```python
from build123d import *

# Parameters (mm, degrees)
SKETCH1_R           = 1.5
BOSS_EXTRUDE1_DEPTH = 222.5


with BuildPart() as part:
    # Sketch1 → Boss-Extrude1 (new body)
    with BuildSketch(Plane.XY):
        with BuildLine():
            Line((0.997149379, -0.010991612), (4.197149379, -0.010991612))
            ThreePointArc((4.197149379, -0.010991612), (4.409281413, 0.076876353), (4.497149379, 0.289008388))
            Line((4.497149379, 0.289008388), (4.497149379, 0.689008388))
            ThreePointArc((4.497149379, 0.689008388), (4.409281413, 0.901140422), (4.197149379, 0.989008388))
            Line((4.197149379, 0.989008388), (3.197149379, 0.989008388))
            ThreePointArc((3.197149379, 0.989008388), (2.985017344, 1.076876353), (2.897149379, 1.289008388))
            Line((2.897149379, 1.289008388), (2.897149379, 2.057637538))
            ThreePointArc((2.897149379, 2.057637538), (2.920422177, 2.174637797), (2.9866975, 2.273825827))
            Line((2.9866975, 2.273825827), (4.61806835, 3.905196677))
            ThreePointArc((4.61806835, 3.905196677), (4.71725638, 3.971472), (4.834256639, 3.994744798))
            Line((4.834256639, 3.994744798), (10.171514939, 3.994744798))
            ThreePointArc((10.171514939, 3.994744798), (10.288515198, 3.971472), (10.387703228, 3.905196677))
            Line((10.387703228, 3.905196677), (12.019074078, 2.273825827))
            ThreePointArc((12.019074078, 2.273825827), (12.085349401, 2.174637797), (12.1086222, 2.057637538))
            Line((12.1086222, 2.057637538), (12.1086222, 1.289008388))
            ThreePointArc((12.1086222, 1.289008388), (12.020754234, 1.076876353), (11.8086222, 0.989008388))
            Line((11.8086222, 0.989008388), (10.797149379, 0.989008388))
            ThreePointArc((10.797149379, 0.989008388), (10.585017344, 0.901140422), (10.497149379, 0.689008388))
            Line((10.497149379, 0.689008388), (10.497149379, 0.289008388))
            ThreePointArc((10.497149379, 0.289008388), (10.585017344, 0.076876353), (10.797149379, -0.010991612))
            Line((10.797149379, -0.010991612), (13.997149379, -0.010991612))
            ThreePointArc((13.997149379, -0.010991612), (14.70425616, 0.281901607), (14.997149379, 0.989008388))
            Line((14.997149379, 0.989008388), (14.997149379, 4.189008388))
            ThreePointArc((14.997149379, 4.189008388), (14.909281413, 4.401140422), (14.697149379, 4.489008388))
            Line((14.697149379, 4.489008388), (14.305261888, 4.489008388))
            ThreePointArc((14.305261888, 4.489008388), (14.093129854, 4.401140422), (14.005261888, 4.189008388))
            Line((14.005261888, 4.189008388), (14.005261888, 3.189008388))
            ThreePointArc((14.005261888, 3.189008388), (13.917393922, 2.976876353), (13.705261888, 2.889008388))
            Line((13.705261888, 2.889008388), (12.936632738, 2.889008388))
            ThreePointArc((12.936632738, 2.889008388), (12.819632479, 2.912281186), (12.720444449, 2.978556509))
            Line((12.720444449, 2.978556509), (11.089073599, 4.609927359))
            ThreePointArc((11.089073599, 4.609927359), (11.006246661, 4.70520219), (10.969948855, 4.826115648))
            Line((10.969948855, 4.826115648), (10.969948855, 10.163373948))
            ThreePointArc((10.969948855, 10.163373948), (11.00546556, 10.284783861), (11.087867966, 10.380761184))
            Line((11.087867966, 10.380761184), (12.719238816, 12.012132034))
            ThreePointArc((12.719238816, 12.012132034), (12.81656582, 12.07716386), (12.93137085, 12.1))
            Line((12.93137085, 12.1), (13.7, 12.1))
            ThreePointArc((13.7, 12.1), (13.912132034, 12.012132034), (14, 11.8))
            Line((14, 11.8), (14, 10.8))
            ThreePointArc((14, 10.8), (14.087867966, 10.587867966), (14.3, 10.5))
            Line((14.3, 10.5), (14.697149379, 10.5))
            ThreePointArc((14.697149379, 10.5), (14.909281413, 10.587867966), (14.997149379, 10.8))
            Line((14.997149379, 10.8), (14.997149379, 13.989008388))
            ThreePointArc((14.997149379, 13.989008388), (14.70425616, 14.696115169), (13.997149379, 14.989008388))
            Line((13.997149379, 14.989008388), (10.797149379, 14.989008388))
            ThreePointArc((10.797149379, 14.989008388), (10.585017344, 14.901140422), (10.497149379, 14.689008388))
            Line((10.497149379, 14.689008388), (10.497149379, 14.289008388))
            ThreePointArc((10.497149379, 14.289008388), (10.585017344, 14.076876353), (10.797149379, 13.989008388))
            Line((10.797149379, 13.989008388), (11.798829534, 13.989008388))
            ThreePointArc((11.798829534, 13.989008388), (12.010961569, 13.901140422), (12.098829534, 13.689008388))
            Line((12.098829534, 13.689008388), (12.098829534, 12.916322983))
            ThreePointArc((12.098829534, 12.916322983), (12.075993394, 12.801517953), (12.010961569, 12.704190949))
            Line((12.010961569, 12.704190949), (10.379590719, 11.072820099))
            ThreePointArc((10.379590719, 11.072820099), (10.282263714, 11.007788273), (10.167458684, 10.984952133))
            Line((10.167458684, 10.984952133), (4.830200384, 10.984952133))
            ThreePointArc((4.830200384, 10.984952133), (4.715395355, 11.007788273), (4.61806835, 11.072820099))
            Line((4.61806835, 11.072820099), (2.9866975, 12.704190949))
            ThreePointArc((2.9866975, 12.704190949), (2.920422177, 12.803378979), (2.897149379, 12.920379238))
            Line((2.897149379, 12.920379238), (2.897149379, 13.689008388))
            ThreePointArc((2.897149379, 13.689008388), (2.985017344, 13.901140422), (3.197149379, 13.989008388))
            Line((3.197149379, 13.989008388), (4.197149379, 13.989008388))
            ThreePointArc((4.197149379, 13.989008388), (4.409281413, 14.076876353), (4.497149379, 14.289008388))
            Line((4.497149379, 14.289008388), (4.497149379, 14.689008388))
            ThreePointArc((4.497149379, 14.689008388), (4.409281413, 14.901140422), (4.197149379, 14.989008388))
            Line((4.197149379, 14.989008388), (0.997149379, 14.989008388))
            ThreePointArc((0.997149379, 14.989008388), (0.290042597, 14.696115169), (-0.002850621, 13.989008388))
            Line((-0.002850621, 13.989008388), (-0.002850621, 10.789008388))
            ThreePointArc((-0.002850621, 10.789008388), (0.085017344, 10.576876353), (0.297149379, 10.489008388))
            Line((0.297149379, 10.489008388), (0.697149379, 10.489008388))
            ThreePointArc((0.697149379, 10.489008388), (0.909281413, 10.576876353), (0.997149379, 10.789008388))
            Line((0.997149379, 10.789008388), (0.997149379, 11.790199043))
            ThreePointArc((0.997149379, 11.790199043), (1.085017344, 12.002331078), (1.297149379, 12.090199043))
            Line((1.297149379, 12.090199043), (2.057928823, 12.090199043))
            ThreePointArc((2.057928823, 12.090199043), (2.174143192, 12.067250491), (2.272911478, 12.001849869))
            Line((2.272911478, 12.001849869), (3.912132034, 10.380761184))
            ThreePointArc((3.912132034, 10.380761184), (3.97928656, 10.281159192), (4.002885789, 10.163373948))
            Line((4.002885789, 10.163373948), (4.002885789, 4.826115648))
            ThreePointArc((4.002885789, 4.826115648), (3.979612991, 4.709115389), (3.913337668, 4.609927359))
            Line((3.913337668, 4.609927359), (2.281966818, 2.978556509))
            ThreePointArc((2.281966818, 2.978556509), (2.182778788, 2.912281186), (2.065778529, 2.889008388))
            Line((2.065778529, 2.889008388), (1.297149379, 2.889008388))
            ThreePointArc((1.297149379, 2.889008388), (1.085017344, 2.976876353), (0.997149379, 3.189008388))
            Line((0.997149379, 3.189008388), (0.997149379, 4.189008388))
            ThreePointArc((0.997149379, 4.189008388), (0.909281413, 4.401140422), (0.697149379, 4.489008388))
            Line((0.697149379, 4.489008388), (0.297149379, 4.489008388))
            ThreePointArc((0.297149379, 4.489008388), (0.085017344, 4.401140422), (-0.002850621, 4.189008388))
            Line((-0.002850621, 4.189008388), (-0.002850621, 0.989008388))
            ThreePointArc((-0.002850621, 0.989008388), (0.290042597, 0.281901607), (0.997149379, -0.010991612))
        make_face()
        with Locations((7.5, 7.5)):
            Circle(SKETCH1_R, mode=Mode.SUBTRACT)
    extrude(amount=BOSS_EXTRUDE1_DEPTH)


solid = part.part
```
Source: CAD feature listing. Evaluate the final solid. Frame: model axes, mm. A direction names the side the tool comes from. Coordinates: 2 decimals unless noted, no trailing zeros. Put each result on its own line as item: value. Start each with the question number.
1) Contact query for a flat-ended pin moving along its axis: pin 1 Ø2.5 at (x, y) = (7.5, 7.5) entering from -Z. Output: stop coordinate, or through.
2) Reachability of faces 1 (the face through (10.97, 7, 110)), 2 (the face through (8, 10.985, 110)), 3 (the face through (7.4, 9.3, 0)) from +Z, -Z, +X, -X, +Y, -Y: full face, straight path, thin tool, end or side. Return the list, or none.
3) Ray query, L1, parallel to Y at x = 7.5, z = 107; L2, parallel to X at y = 11.5, z = 163; L3, parallel to X at y = 12.75, z = 101. Return the intervals inside material, ascending. Write a range as from..to.
4) Pull-direction query (Y, two-part tool) for faces 4 (the face through (7, 3.995, 110)), 5 (the face through (7.4, 9.3, 222.5)), 6 (the face through (4.003, 8, 110)); classes: pulls with the +Y half, pulls with the -Y half, needs draft (parallel to the pull), parting line crosses it, or undercut.
The answers:
1. pin 1: passes through
2. face 1: +Z, -Z, +X
2. face 2: +Z, -Z, +Y
2. face 3: -Z, +X, -X, +Y, -Y
3. L1: y = 3.99..6, 9..10.98
3. L2: x = 0..1, 2.78..4.19, 10.81..12.21, 14..15
3. L3: x = 0..2.95, 12.05..15
4. face 4: pulls with the -Y half
4. face 5: needs draft
4. face 6: undercut
